The listing builds one solid part. Answer for the finished solid, in the listing's coordinates (mm). A direction names the side the tool comes from. Coordinates: 2 decimals unless noted, no trailing zeros. Order: outer loops, then holes, each group sorted by start corner. A loop starts at its lowest first (then second) coordinate and runs counter-clockwise, first axis right, second up. Notation, with made-up numbers: (-29.5, -21.75) -> (-19.5, -21.75) arc R30 cw to (-19.5, 7.25) -> close; hole circle Ø3 at (1, 65.25). An arc over 180 degrees is marked (long way). Return JSON: item names as keys, results as strings.
```python
from build123d import *

# Parameters (mm, degrees)
SKETCH1_W           = 80
SKETCH1_H           = 50.725
SKETCH1_H_2         = 101.6
SKETCH1_R           = 3.25
BOSS_EXTRUDE1_DEPTH = 10
SKETCH1_3_W         = 80
SKETCH1_3_H         = 50.725
BOSS_EXTRUDE2_DEPTH = 25.4
SKETCH2_R           = 2
CUT_EXTRUDE1_DEPTH  = 74.7143134


with BuildPart() as part:
    # Sketch1 → Boss-Extrude1 (new body)
    # profile 1 of 2: a face of its own
    with BuildSketch(Plane(origin=(0, 0, 0), x_dir=(1, 0, 0), z_dir=(0, 1, 0))):
        Rectangle(SKETCH1_W, SKETCH1_H)
    # profile 2 of 2: a face of its own
    with BuildSketch(Plane(origin=(0, 0, 0), x_dir=(1, 0, 0), z_dir=(0, 1, 0))):
        Rectangle(SKETCH1_W, SKETCH1_H_2)
        with Locations(Location((-27.28125, 38.08125, 0), (0, 0, 270))):
            Circle(SKETCH1_R, mode=Mode.SUBTRACT)
        with Locations(Location((27.28125, 38.08125, 0), (0, 0, 270))):
            Circle(SKETCH1_R, mode=Mode.SUBTRACT)
        with Locations(Location((-27.28125, -38.08125, 0), (0, 0, 270))):
            Circle(SKETCH1_R, mode=Mode.SUBTRACT)
        with Locations(Location((27.28125, -38.08125, 0), (0, 0, 270))):
            Circle(SKETCH1_R, mode=Mode.SUBTRACT)
    extrude(amount=BOSS_EXTRUDE1_DEPTH)

    # Sketch1_3 → Boss-Extrude2 (add)
    with BuildSketch(Plane(origin=(0, 0, 0), x_dir=(1, 0, 0), z_dir=(0, 1, 0))):
        Rectangle(SKETCH1_3_W, SKETCH1_3_H)
    extrude(amount=-BOSS_EXTRUDE2_DEPTH)

    # Sketch2 → Cut-Extrude1 (cut, through all)
    with BuildSketch(Plane(origin=(0, 10, 0), x_dir=(1, 0, 0), z_dir=(0, 1, 0))):
        with Locations(Location((-28.575, -13.97, 0), (0, 0, 270))):
            Circle(SKETCH2_R)
        with Locations(Location((28.575, 13.97, 0), (0, 0, 270))):
            Circle(SKETCH2_R)
    extrude(amount=-CUT_EXTRUDE1_DEPTH, mode=Mode.SUBTRACT)


solid = part.part
```
Item 1: Which of the six approach directions +Z, -Z, +X, -X, +Y, -Y give full straight-line access (tool end or side, diameter ignored) to faces 1 (the flat face through (-1, 0, 38)), 2 (the flat face through (-1, -13, -25.362)), 3 (the cylindrical face through (-29.26, 4.93, -40.66))?
Answer list:
{"face 1": "+Z, +X, -X, -Y", "face 2": "-Z, +X, -X, -Y", "face 3": "+Y, -Y"}
Item 2: The part is cut by section A-A on z = -13.97. Determine the outline of the cut face in (x, y) (3 decimals).
Answer list:
{"outline": "(-40, -25.4) -> (26.575, -25.4) -> (26.575, 10) -> (-40, 10) -> close; (30.575, -25.4) -> (40, -25.4) -> (40, 10) -> (30.575, 10) -> close"}
Item 3: The part is cut by section B-B on x = 2. Determine the outline of the cut face in (y, z).
Answer list:
{"outline": "(-25.4, -25.36) -> (0, -25.36) -> (0, -50.8) -> (10, -50.8) -> (10, 50.8) -> (0, 50.8) -> (0, 25.36) -> (-25.4, 25.36) -> close"}
Item 4: Determine the mould class of faces 4 (the flat face through (-1, 10, -1)), 5 (the flat face through (-1, -13, 25.362)), 6 (the flat face through (-1, 5, -50.8)), 7 (the cylindrical face through (25.3, 4.93, -40.66)) for opening direction Z: pulls with the +Z half, pulls with the -Z half, needs draft (parallel to the pull), parting line crosses it, or undercut.
Answer list:
{"face 4": "needs draft", "face 5": "pulls with the +Z half", "face 6": "pulls with the -Z half", "face 7": "undercut"}
Item 5: Find the intervals of material crossed by probe 1 along X at (y, z) = (-14.5, 13.97) (3 decimals); probe 2 along Y at (x, z) = (2, 35); probe 3 along Z at (x, y) = (16.5, -8.5), in increasing order.
Answer list:
{"probe 1": "-40 to -30.575, -26.575 to 40", "probe 2": "0 to 10", "probe 3": "-25.36 to 25.36"}
Item 6: The part is cut by section C-C on y = 3. Determine the outline of the cut face in (x, z) (3 decimals).
Answer list:
{"outline": "(-40, -50.8) -> (40, -50.8) -> (40, 50.8) -> (-40, 50.8) -> close; hole circle Ø4 at (-28.575, 13.97); hole circle Ø6.5 at (-27.281, -38.081); hole circle Ø6.5 at (-27.281, 38.081); hole circle Ø6.5 at (27.281, -38.081); hole circle Ø6.5 at (27.281, 38.081); hole circle Ø4 at (28.575, -13.97)"}
Item 7: The part is cut by section D-D on y = -15. Determine the outline of the cut face in (x, z) (1 decimal), plus the area to 3 significant figures.
Answer list:
{"outline": "(-40, -25.4) -> (40, -25.4) -> (40, 25.4) -> (-40, 25.4) -> close; hole circle Ø4 at (-28.6, 14); hole circle Ø4 at (28.6, -14)", "area": "4,030 mm2"}
Item 8: Flat-ended cylindrical pins translate along their axes: pin 1 (1 mm diameter, centred on x = -13, y = -13.5, fed in from -Z); pin 2 (4 mm diameter, centred on x = 21.5, y = -13.5, fed in from +Z); pin 3 (6 mm diameter, centred on x = -27.28, z = 38.08, fed in from -Y); pin 4 (6 mm diameter, centred on x = 6.5, y = -1, fed in from +Z). Find the tip coordinate at first contact, or state that the pin passes through.
Answer list:
{"pin 1": "z = -25.36", "pin 2": "z = 25.36", "pin 3": "through", "pin 4": "z = 50.8"}
